from build123d import *

# Parameters (mm, degrees)
SKETCH_1_W          = 45
SKETCH_1_H          = 40
SKETCH_1_W_2        = 30
SKETCH_1_H_2        = 30
EXTRUDE_2_DEPTH     = 3
CUT_EXTRUDE_2_DEPTH = 30
SKETCH_3_W          = 5
SKETCH_3_H          = 5
SKETCH_3_R          = 1.55
EXTRUDE_3_DEPTH     = 5


with BuildPart() as part:
    # 草图1 → 凸台-拉伸2 (new body)
    with BuildSketch(Plane(origin=(0, 0, 0), x_dir=(1, 0, 0), z_dir=(0, 1, 0))):
        Rectangle(SKETCH_1_W, SKETCH_1_H)
        with Locations((-2.5, 0)):
            Rectangle(SKETCH_1_W_2, SKETCH_1_H_2, mode=Mode.SUBTRACT)
    extrude(amount=EXTRUDE_2_DEPTH)

    # 草图2 → 切除-拉伸2 (cut)
    with BuildSketch(Plane.XY.offset(-15)):
        Polygon((12.5, 0), (15.5, 0), (15.5, 2.196152423), (12.5, 3), align=None)
    extrude(amount=CUT_EXTRUDE_2_DEPTH, mode=Mode.SUBTRACT)

    # 草图3 → 凸台-拉伸3 (add)
    with BuildSketch(Plane.XY.offset(20)):
        with Locations((1.5, 5.5)):
            Rectangle(SKETCH_3_W, SKETCH_3_H)
        with Locations((1.5, 5.5)):
            Circle(SKETCH_3_R, mode=Mode.SUBTRACT)
    extrude_3 = extrude(amount=-EXTRUDE_3_DEPTH)

    # 镜向2: 凸台-拉伸3 across plane
    add(extrude_3.mirror(Plane(origin=(0, 0, 0), x_dir=(1, 0, 0), z_dir=(0, 0, -1))))


solid = part.part
For this review, take the finished solid that the model builds, in its own axes (mm). A direction names the side the tool comes from. Coordinates: 2 decimals unless noted, no trailing zeros. Loops run counter-clockwise (first coordinate to the right, second up) from the corner with the lowest first, then second, coordinate; pieces in that order, holes last. Notation, with made-up numbers: (29.25, 56) - (34.25, 56) arc R20 cw to (34.25, 84) - close; hole circle Ø7 at (-35.75, 83.25). An arc over 180 degrees is marked (long way). Use a Markdown table: item, result. Add a question column.
Item 1: We need section D-D (x = 1.5). Give the boundary of the cut face in (y, z).
Item 2: We need section C-C (x = -5.5). Give the boundary of the cut face in (y, z).
Item 3: We need section A-A (z = -3.5). Give the boundary of the cut face in (x, y), and give its area (3 significant figures).
Item 4: Mouldability with a two-part tool opening along Y and no side actions: class faces 1 (the face through (1.298, 7.037, -17.535)), 2 (the face through (0, 0, 17)), 3 (the face through (15.5, 1, 0)), 4 (the face through (1.298, 7.037, 17.535)) as pulls with the +Y half, pulls with the -Y half, needs draft (parallel to the pull), parting line crosses it, or undercut.
Item 5: Insertion check: pin 1 Ø9 at (x, z) = (16.5, 3.5) entering from +Y; pin 2 Ø1.5 at (y, z) = (4.5, -18.5) entering from -X; pin 3 Ø4 at (y, z) = (6, 17.5) entering from +X. Each pin has a flat end and moves straight along its axis. Give the tip position at first contact, or say it passes through.
Item 6: Tool access review of faces 5 (the face through (-17.5, 1, 0)), 6 (the face through (14, 2.6, -0.2)), 7 (the face through (-19, 3, 0)), 8 (the face through (15, 3, 0)): name each direction out of +Z, -Z, +X, -X, +Y, -Y from which nothing blocks a thin tool from reaching the whole face with its end or side.
Item 7: For line 1 (Z direction, x = -4.5, y = 2.5); line 2 (Y direction, x = 1.5, z = 18.3); line 3 (X direction, y = 2, z = 5), list the stretches that pass through material, from the lowest coordinate up.
Item 8: We need section B-B (y = 5.5). Give the boundary of the cut face in (x, z), and give its area (3 significant figures).
Results list:
| question | item | result |
|---|---|---|
| 1 | outline | (0, -20) - (3.95, -20) - (3.95, -15) - (0, -15) - close; (0, 15) - (3.95, 15) - (3.95, 20) - (0, 20) - close; (7.05, -20) - (8, -20) - (8, -15) - (7.05, -15) - close; (7.05, 15) - (8, 15) - (8, 20) - (7.05, 20) - close |
| 2 | outline | (0, -20) - (3, -20) - (3, -15) - (0, -15) - close; (0, 15) - (3, 15) - (3, 20) - (0, 20) - close |
| 3 | outline | (-22.5, 0) - (-17.5, 0) - (-17.5, 3) - (-22.5, 3) - close; (12.5, 3) - (15.5, 2.2) - (15.5, 0) - (22.5, 0) - (22.5, 3) - close |
| 3 | area | 37.2 mm^2 |
| 4 | face 1 | undercut |
| 4 | face 2 | pulls with the -Y half |
| 4 | face 3 | needs draft |
| 4 | face 4 | undercut |
| 5 | pin 1 | stops at y = 3 |
| 5 | pin 2 | stops at x = -1 |
| 5 | pin 3 | stops at x = 4 |
| 6 | face 5 | +Y, -Y |
| 6 | face 6 | -Y |
| 6 | face 7 | +Z, -Z, -X, +Y |
| 6 | face 8 | +Z, -Z, +X, +Y |
| 7 | line 1 | z = -20 to -15, 15 to 20 |
| 7 | line 2 | y = 0 to 3.95, 7.05 to 8 |
| 7 | line 3 | x = -22.5 to -17.5, 15.5 to 22.5 |
| 8 | outline | (-1, -20) - (-0.05, -20) - (-0.05, -15) - (-1, -15) - close; (-1, 15) - (-0.05, 15) - (-0.05, 20) - (-1, 20) - close; (3.05, -20) - (4, -20) - (4, -15) - (3.05, -15) - close; (3.05, 15) - (4, 15) - (4, 20) - (3.05, 20) - close |
| 8 | area | 19.0 mm^2 |
